For this review, take the finished solid that the model builds, in its own axes (mm). Face numbers are marked on the shaded views. A direction names the side the tool comes from. Round coordinates to 2 decimals unless told otherwise and drop trailing zeros. One line per question, with ' | ' between items.
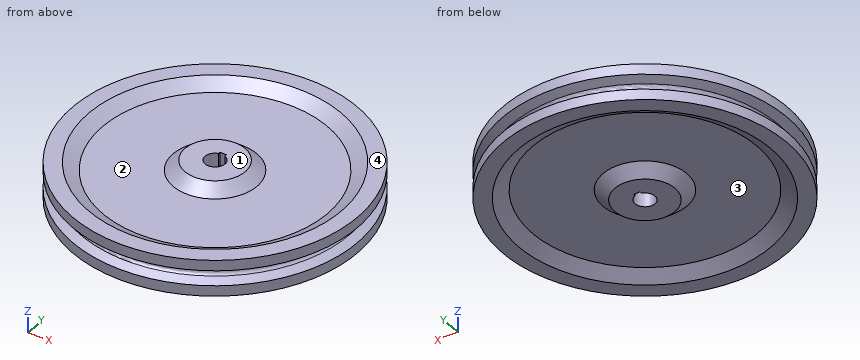
```python
from build123d import *
from build123d.topology import SkipClean

# Parameters (mm, degrees)
ESQUISSE2_R             = 25
ENL_V_MAT_EXTRU_1_DEPTH = 512.908194894
ESQUISSE3_W             = 16
ESQUISSE3_H             = 8.6
ENL_V_MAT_EXTRU_2_DEPTH = 512.908194894


with BuildPart() as part:
    # Esquisse1 → Révolution1 (revolve)
    with BuildSketch(Plane(origin=(0, 0, 0), x_dir=(0, 0, -1), z_dir=(1, 0, 0)), mode=Mode.PRIVATE) as r_volution1_sk:
        with BuildLine():
            Line((0, 0), (-50, 0))
            Line((-50, 0), (-50, 75))
            Line((-50, 75), (-25, 104.793839815))
            Line((-25, 104.793839815), (-25, 280.358983849))
            Line((-25, 280.358983849), (-45, 315))
            Line((-45, 315), (-45, 355))
            Line((-45, 355), (-18.820962226, 355))
            Line((-18.820962226, 355), (-9.700735091, 332.98182396))
            ThreePointArc((-9.700735091, 332.98182396), (-5.833487447, 328.269569071), (0, 326.5))
            Line((0, 326.5), (0, 0))
        make_face()
    r_volution1 = revolve(r_volution1_sk.sketch.rotate(Axis((0, 0, 0), (0, 0, 1)), 90), axis=Axis((0, 0, 0), (0, 0, 1)))

    # Symétrie1: Révolution1 across plane
    with SkipClean():  # the faces are left unmerged after this step: merging them gives an invalid solid
        add(r_volution1.mirror(Plane(origin=(0, 326.5, 0), x_dir=(1, 0, 0), z_dir=(0, 0, -1))))

    # Esquisse2 → Enlèv. mat.-Extru.1 (cut, through all)
    with SkipClean():  # the faces are left unmerged after this step: merging them gives an invalid solid
        with BuildSketch(Plane.XY.offset(50)):
            Circle(ESQUISSE2_R)
        extrude(amount=-ENL_V_MAT_EXTRU_1_DEPTH, mode=Mode.SUBTRACT)

    # Esquisse3 → Enlèv. mat.-Extru.2 (cut, through all)
    with SkipClean():  # the faces are left unmerged after this step: merging them gives an invalid solid
        with BuildSketch(Plane.XY.offset(50)):
            with Locations((0, 25)):
                Rectangle(ESQUISSE3_W, ESQUISSE3_H)
        extrude(amount=-ENL_V_MAT_EXTRU_2_DEPTH, mode=Mode.SUBTRACT)


solid = part.part
```
(1) For the marked faces 1 and 2, list the 3-axis set-ups (+Z, -Z, +X, -X, +Y, -Y) from which the entire face can be reached by the end or side of a thin tool; tool diameter is ignored.
Output values:
face 1: +Z, +X, -X, +Y, -Y | face 2: +Z
(2) Insertion check: pin 1 (4.5 mm diameter, centred on y = 25.5, z = -21.5, fed in from +X); pin 2 (6 mm diameter, centred on x = 71.5, y = 109.5, fed in from -Z); pin 3 (10 mm diameter, centred on y = -246.5, z = -38.5, fed in from -X). Each pin has a flat end and moves straight along its axis. Give the tip position at first contact, or say it passes through.
Output values:
pin 1: x = 354.24 | pin 2: z = -25 | pin 3: x = -260.2
(3) Mouldability with a two-part tool opening along X and no side actions: class the marked faces 3 and 4 as released by +X, released by -X, zero draft, split by the parting line, or undercut.
Output values:
face 3: undercut | face 4: zero draft
(4) For probe 1 along Y at (x, z) = (0, -21); probe 2 along Z at (x, y) = (262, 13); probe 3 along X at (y, z) = (164.5, 36.5), list the stretches that pass through material, from the lowest coordinate up. Write a range as [from, to].
Output values:
probe 1: [-355, -25], [29.3, 355] | probe 2: [-25, 25] | probe 3: [-314.59, -251.21], [251.21, 314.59]
